Check sheet for the modelled part. Datum: model origin and axes. Units: mm. A direction names the side the tool comes from. Coordinates: 2 decimals unless noted, no trailing zeros. Write each loop counter-clockwise with the first axis right and the second up, starting at its lowest first coordinate (ties: lowest second). Pieces come first, ordered by that corner, then holes. Notation, with made-up numbers: M 79.25,1.5 L 126.25,1.5 A28 cw 126.25,22.5 Z; hole C 47,-3.5 d2. An arc over 180 degrees is marked long. Answer as CSV lines item,"result". Start each with the question number.
Q1. Access from +Z, -Z, +X, -X, +Y, -Y to the whole of each face (thin tool, end or side, straight path). Record for faces 1 (the flat face through (3, -6.617, 21)), 2 (the flat face through (17.844, 12, 21)).
Q2. Thickness scan on line 1 along X through (y, z) = (-4.95, 35.5); line 2 along Y through (x, z) = (18.6, 21.5); line 3 along X through (y, z) = (-4, 7). Record the ranges inside material, lowest first. Write a range as from..to.
Q3. Depth check by flat-ended pin: pin 1 Ø9.5 at (y, z) = (22, 28.5) entering from -X; pin 2 Ø3.5 at (x, z) = (-7.16, 21.5) entering from +Y; pin 3 Ø2.5 at (x, z) = (-7.16, 35.5) entering from +Y. Enter the tip coordinate at first touch or a pass-through.
Q4. Sectioned sample at C-C, the plane x = 7. Record the cut outline in (y, z).
Q5. Sectioned sample at A-A, the plane z = 21.5. Record the cut outline in (x, y), then the cut area to 3 significant figures.
Q6. Sectioned sample at B-B, the plane z = 7.5. Record the cut outline in (x, y), then the cut area to 3 significant figures.
Q7. Sectioned sample at D-D, the plane z = 16. Record the cut outline in (x, y), then the cut area to 3 significant figures.
Q8. Mould release check, pull along Z, two halves, no side actions. Record for faces 3 (the cylindrical face through (-14.554, -5.138, 42.43)), 4 (the cylindrical face through (-6.24, -5.1, 36.69)), 5 (the cylindrical face through (-14.585, -5.138, 0.601)): pulls with the +Z half, pulls with the -Z half, needs draft (parallel to the pull), parting line crosses it, or undercut.
Autodesk Inventor part; units mm, degrees
ref_plane "YZ Plane" through (0, 0, 0) normal (1, 0, 0) x (0, 1, 0)
ref_plane "XZ Plane" through (0, 0, 0) normal (0, 1, 0) x (-1, 0, 0)
ref_plane "XY Plane" through (0, 0, 0) normal (0, 0, 1) x (1, 0, 0)
sketch "Szkic1" plane through (0, 0, 0) normal (0, 0, 1) x (1, 0, 0)
  line L0 (-15.1556, -3.6171) -> (-15.1556, -6.6171)
  line L1 (-15.1556, -6.6171) -> (20.8444, -6.6171)
  line L2 (20.8444, -6.6171) -> (20.8444, 40.3829)
  line L3 (20.8444, 40.3829) -> (17.8444, 40.3829)
  line L4 (17.8444, 40.3829) -> (17.8444, -3.6171)
  line L5 (17.8444, -3.6171) -> (-15.1556, -3.6171)
  point P0 (0, 0)
  dimension "d0" = 3
  dimension "d1" = 36
  dimension "d2" = 47
  dimension "d3" = 3
extrude "Wyciągnięcie proste1" add sketch "Szkic1" along normal blind 43
fillet "Zaokrąglenie1" radius 3 1 edges at (17.8444, -3.6171, 21.5)
fillet "Zaokrąglenie2" radius 2 2 edges at (-15.1556, -5.1171, 0) (-15.1556, -5.1171, 43)
sketch "Szkic3" plane through (20.8444, -6.6171, 0) normal (0, -1, 0) x (1, 0, 0)
  arc A0 (-34, 43) -> (-36, 41) centre (-34, 41) ccw
  line L0 (-36, 2) -> (-36, 41)
  arc A1 (-36, 2) -> (-34, 0) centre (-34, 2) ccw
  line L1 (-34, 0) -> (0, 0)
  line L2 (0, 0) -> (0, 43)
  line L3 (-34, 43) -> (0, 43)
  point P0 (-20.8444, 0)
  point P1 (-28, 35.5)
  point P2 (-8, 35.5)
  point P3 (-28, 7.5)
  point P4 (-8, 7.5)
  dimension "d40" = 20
  dimension "d41" = 20
  dimension "d42" = 36
  dimension "d43" = 8
  dimension "d44" = 8
  dimension "d45" = 7.5
  dimension "d46" = 7.5
  dimension "d47" = 7.5
  dimension "d48" = 7.5
hole "Otwór3" at (-7.1556, -6.6171, 35.5) at (12.8444, -6.6171, 35.5) at (-7.1556, -6.6171, 7.5) at (12.8444, -6.6171, 7.5) direction (0, 1, 0) diameter 3 end through all
sketch "Szkic4" plane through (20.8444, -6.6171, 0) normal (1, 0, 0) x (0, 0, -1)
  line L0 (0, 0) -> (0, 47)
  line L1 (0, 47) -> (-43, 47)
  line L2 (-43, 0) -> (-43, 47)
  line L3 (0, 0) -> (-43, 0)
  line L4 (0, 3) -> (-43, 3)
  circle A0 centre (-21.5, 27.5) radius 10
  line L5 (-43, 3) -> (-30.6773, 31.472)
  line L6 (0, 3) -> (-12.3227, 31.472)
  point P0 (0, 6.6171)
  dimension "d57" = 43
  dimension "d58" = 21.5
  dimension "d59" = 27.5
  dimension "d60" = 20
extrude "Wyciągnięcie proste4" cut sketch "Szkic4" against normal blind 10 contours L6 A0 L5 L2 L1 L0
hole "Otwór4" at (20.8444, 20.8829, 21.5) direction (-1, 0, 0) diameter 4 end through all
sketch "Szkic5" plane through (-15.1556, -3.6171, 41) normal (0, 1, 0) x (1, 0, 0)
  circle A0 centre (28, 5.5) radius 1.5
  circle A1 centre (28, 33.5) radius 1.5
  circle A2 centre (28, 5.5) radius 3.1
  circle A3 centre (28, 33.5) radius 1.5
  circle A4 centre (28, 33.5) radius 3.1
  point P0 (15.1556, 41)
  dimension "d70" = 6.2
  dimension "d71" = 6.2
extrude "Wyciągnięcie proste5" cut sketch "Szkic5" along normal blind 10
sketch "Szkic6" plane through (20.8444, -6.6171, 0) normal (0, -1, 0) x (1, 0, 0)
  circle A0 centre (-28, 7.5) radius 1.5
  circle A1 centre (-28, 35.5) radius 1.5
  circle A2 centre (-8, 35.5) radius 1.5
  circle A3 centre (-8, 7.5) radius 1.5
  arc A4 (-34, 43) -> (-36, 41) centre (-34, 41) ccw
  line L0 (-36, 2) -> (-36, 41)
  arc A5 (-36, 2) -> (-34, 0) centre (-34, 2) ccw
  line L1 (-34, 0) -> (0, 0)
  line L2 (0, 0) -> (0, 43)
  line L3 (-34, 43) -> (0, 43)
  point P0 (-20.8444, 0)
  point P1 (-28, 21.5)
  point P2 (-8, 21.5)
  dimension "d74" = 14
  dimension "d75" = 14
  dimension "d76" = 14
  dimension "d77" = 14
hole "Otwór5" at (-7.1556, -6.6171, 21.5) at (12.8444, -6.6171, 21.5) direction (0, 1, 0) diameter 3 end through all
properties part number "CNCM_ALU_X_Axis_Idler_Mounting_Bracket"
Output:
1,face 1,"+Z, -Z, +X, -X, -Y"
1,face 2,"+Z, -Z, -X, +Y"
2,line 1,"x = -15.16..-8.66, -5.66..11.34, 14.34..20.84"
2,line 2,"y = -6.62..18.88, 22.88..30.88"
2,line 3,"x = -15.16..-8.57, -5.74..11.43, 14.26..20.84"
3,pin 1,"stops at x = 17.84"
3,pin 2,"stops at y = -3.62"
3,pin 3,"passes through"
4,outline,"M -6.62,0 L -3.62,0 L -3.62,43 L -6.62,43 Z"
5,outline,"M -15.16,-6.62 L -8.66,-6.62 L -8.66,-3.62 L -15.16,-3.62 Z; M -5.66,-6.62 L 11.34,-6.62 L 11.34,-3.62 L -5.66,-3.62 Z; M 14.34,-6.62 L 20.84,-6.62 L 20.84,18.88 L 17.84,18.88 L 17.84,-0.62 A3 cw 14.84,-3.62 L 14.34,-3.62 Z; M 17.84,22.88 L 20.84,22.88 L 20.84,30.88 L 17.84,30.88 Z"
5,area,"183 mm^2"
6,outline,"M -15.16,-6.62 L -8.66,-6.62 L -8.66,-3.62 L -15.16,-3.62 Z; M -5.66,-6.62 L 11.34,-6.62 L 11.34,-3.62 L -5.66,-3.62 Z; M 14.34,-6.62 L 20.84,-6.62 L 20.84,13.71 L 17.84,13.71 L 17.84,-0.62 A3 cw 15.94,-3.41 L 15.94,-3.62 L 14.34,-3.62 Z"
6,area,"144 mm^2"
7,outline,"M -15.16,-6.62 L 20.84,-6.62 L 20.84,29.23 L 17.84,29.23 L 17.84,-0.62 A3 cw 14.84,-3.62 L -15.16,-3.62 Z"
7,area,"208 mm^2"
8,face 3,"pulls with the +Z half"
8,face 4,"undercut"
8,face 5,"pulls with the -Z half"
